Could you check a few things on this model? Use its own coordinates, in mm. A direction names the side the tool comes from. Give positions to 0.01 mm unless a question says otherwise; leave off trailing zeros. Loops run counter-clockwise (first coordinate to the right, second up) from the corner with the lowest first, then second, coordinate; pieces in that order, holes last. Notation, with made-up numbers: M 46,43 L 61,43 A13 ccw 61,58 Z; hole C -13,75 d1. An arc over 180 degrees is marked long. Return JSON: item names as keys, results as strings. Group by question number.
1. For pin 1 (5 mm diameter, centred on x = 4.5, z = 17, fed in from +Y); pin 2 (6 mm diameter, centred on x = -10.65, y = 5.23, fed in from +Z); pin 3 (6 mm diameter, centred on x = -4.5, z = 4, fed in from -Y); pin 4 (1 mm diameter, centred on y = 3, z = 2.5, fed in from -X), each with a flat end and sliding along its axis, tell me the tip position at first contact or that it passes through.
2. For faces 5 (the flat face through (-11, 5, 10.16)), 6 (the flat face through (15, 4, 3.6)), 7 (the flat face through (3, 7.85, 10)), 8 (the flat face through (13.3, 4, 3)), 9 (the flat face through (-10, -7.85, 7)), which set-ups out of +Z, -Z, +X, -X, +Y, -Y let a thin tool reach every point of the face, with its end or its side?
3. If we section it at D-D (x = 6.5): Write out the boundary of the cut face in (y, z).
4. If we section it at C-C (z = 6.5): Write out the boundary of the cut face in (x, y).
5. If we section it at A-A (y = 10.9): Write out the boundary of the cut face in (x, z).
6. If we mould it in two halves opening along X, with no side actions, what happens to faces 1 (the flat face through (-17, 0, 1)), 2 (the flat face through (0, -13.25, 1)), 3 (the flat face through (17, 0, 1)), 4 (the flat face through (-6.2, 0, 10))? For each: +X half, -X half, draft (parallel to the pull), parting line (faces both ways), or undercut.
7. If we section it at B-B (x = 14.4): Write out the boundary of the cut face in (y, z).
8. Please list where these lines run through material, in increasing order: line 1 (Y direction, x = 14.4, z = 1.15); line 2 (Y direction, x = -10.65, z = 11); line 3 (X direction, y = 5.25, z = 10.75).
Autodesk Inventor part; units mm, degrees
ref_plane "YZ Plane" through (0, 0, 0) normal (1, 0, 0) x (0, 1, 0)
ref_plane "XZ Plane" through (0, 0, 0) normal (0, 1, 0) x (-1, 0, 0)
ref_plane "XY Plane" through (0, 0, 0) normal (0, 0, 1) x (1, 0, 0)
sketch "스케치1" plane through (0, 0, 0) normal (0, 0, 1) x (1, 0, 0)
  line L0 (-17, 13.25) -> (17, 13.25)
  line L1 (17, 13.25) -> (17, -13.25)
  line L2 (17, -13.25) -> (-17, -13.25)
  line L3 (-17, -13.25) -> (-17, 13.25)
  line L4 (-17, 13.25) -> (17, -13.25) construction
  line L5 (17, 13.25) -> (-17, -13.25) construction
  circle A0 centre (14.4, 10.9) radius 1.4
  line L6 (0, 0) -> (4.1971, 0)
  line L7 (0, 0) -> (0, 5.4603)
  circle A1 centre (-14.4, 10.9) radius 1.4
  circle A2 centre (14.4, -10.9) radius 1.4
  circle A3 centre (-14.4, -10.9) radius 1.4
  dimension "d0" = 34
  dimension "d1" = 26.5
  dimension "d2" = 28.8
  dimension "d3" = 2.8
  dimension "d4" = 21.8
extrude "돌출1" add sketch "스케치1" along normal blind 1.6
sketch "스케치2" plane through (0, 0, 1.6) normal (0, 0, 1) x (1, 0, 0)
  line L0 (12.6, -7.85) -> (-6.2, -7.85)
  line L1 (-6.2, -7.85) -> (-6.2, 7.85)
  line L2 (-6.2, 7.85) -> (12.6, 7.85)
  line L3 (12.6, 7.85) -> (12.6, -7.85)
  line L4 (12.6, -7.85) -> (-6.2, 7.85) construction
  line L5 (-6.2, -7.85) -> (12.6, 7.85) construction
  line L6 (17, -13.25) -> (17, 13.25)
  point P0 (0, 0)
  point P1 (3.2, 0)
  dimension "d7" = 15.7
  dimension "d8" = 18.8
  dimension "d9" = 4.4
extrude "돌출2" add sketch "스케치2" along normal blind 17.2
sketch "스케치3" plane through (-6.2, 7.85, 1.6) normal (0, 1, 0) x (1, 0, 0)
  line L0 (0, 0) -> (18.8, 0)
  line L1 (0, 0) -> (-1.75, 0)
  line L2 (-1.75, 0) -> (-1.75, -6.84)
  line L3 (-1.75, -6.84) -> (0, -6.84)
  line L4 (0, -6.84) -> (0, 0)
  line L5 (-1.75, 0) -> (-7.75, 0)
  line L6 (-7.75, 0) -> (-7.75, -10.1)
  line L7 (-7.75, -10.1) -> (-1.75, -10.1)
  line L8 (-1.75, -10.1) -> (-1.75, 0)
  line L9 (-7.15, -10.1) -> (-7.75, -6.4)
  line L10 (-0.1, -6.84) -> (-0.1, 0)
  line L11 (23.2, 0) -> (-10.8, 0)
  point P0 (6.2, 1.6)
  point P1 (-1.75, -6.84)
  dimension "d12" = 1.75
  dimension "d13" = 6.84
  dimension "d14" = 6
  dimension "d15" = 10.1
  dimension "d16" = 0.6
  dimension "d17" = 3.7
  dimension "d20" = 0.1
extrude "돌출3" add sketch "스케치3" against normal blind 15.7 contours L10 L3 L2 L1 | L2 L8 L7 L9 L6 L5
sketch "스케치4" plane through (-13.35, 7.85, 11.7) normal (0, 0, 1) x (1, 0, 0)
  line L0 (0, 0) -> (5.4, 0)
  line L1 (0, 0) -> (0, -15.7)
  line L2 (5.4, -15.7) -> (0, -15.7)
  line L3 (5.4, 0) -> (5.4, -15.7)
  line L4 (5.4, 0) -> (5.4, -15.7)
  line L5 (5.4, -7.85) -> (0, -7.85)
  circle A0 centre (2.7, -7.85) radius 1.9
  circle A1 centre (2.7, -13.0833) radius 1.9
  circle A2 centre (2.7, -2.6167) radius 1.9
  circle A3 centre (2.7, -7.85) radius 1.9
  point P0 (13.35, -7.85)
  dimension "d21" = 3.8
  dimension "d24" = 5.2333
  dimension "d27" = 5.2333
extrude "돌출4" cut sketch "스케치4" against normal blind 1.54 contours A0 L5 | L5 A0 | A1 | A2
sketch "스케치5" plane through (0, 0, 1.6) normal (0, 0, 1) x (1, 0, 0)
  line L0 (15.8, 7.85) -> (13.3, 7.85)
  line L1 (13.3, 7.85) -> (13.3, 0.4)
  line L2 (13.3, 0.4) -> (15.8, 0.4)
  line L3 (15.8, 0.4) -> (15.8, 7.85)
  line L4 (17, -13.25) -> (17, 13.25)
  point P0 (0, 0)
  dimension "d32" = 2.5
  dimension "d33" = 7.45
  dimension "d34" = 1.2
extrude "돌출5" add sketch "스케치5" along normal blind 2
chamfer "모따기1" distance 0.5 angle 45 4 edges at (15.8, 7.85, 2.6) (15.8, 0.4, 2.6) (13.3, 7.85, 2.6) (13.3, 0.4, 2.6)
properties part number "릴레이모듈"
Answer:
{
 "1": {"pin 1": "stops at y = 7.85", "pin 2": "stops at z = 11.7", "pin 3": "stops at y = -13.25", "pin 4": "stops at x = -13.95"},
 "2": {"face 5": "+Z", "face 6": "+Z, +X, +Y, -Y", "face 7": "+Z, +X, -X, +Y", "face 8": "+Z, +Y, -Y", "face 9": "+Z, +X, -X, -Y"},
 "3": {"outline": "M -13.25,0 L 13.25,0 L 13.25,1.6 L 7.85,1.6 L 7.85,18.8 L -7.85,18.8 L -7.85,1.6 L -13.25,1.6 Z"},
 "4": {"outline": "M -13.95,-7.85 L -6.3,-7.85 L -6.3,7.85 L -13.95,7.85 Z; M -6.2,-7.85 L 12.6,-7.85 L 12.6,7.85 L -6.2,7.85 Z"},
 "5": {"outline": "M -17,0 L -15.8,0 L -15.8,1.6 L -17,1.6 Z; M -13,0 L 13,0 L 13,1.6 L -13,1.6 Z; M 15.8,0 L 17,0 L 17,1.6 L 15.8,1.6 Z"},
 "6": {"face 1": "-X half", "face 2": "draft", "face 3": "+X half", "face 4": "undercut"},
 "7": {"outline": "M -13.25,0 L -12.3,0 L -12.3,1.6 L -13.25,1.6 Z; M -9.5,0 L 9.5,0 L 9.5,1.6 L 7.85,1.6 L 7.85,3.6 L 0.4,3.6 L 0.4,1.6 L -9.5,1.6 Z; M 12.3,0 L 13.25,0 L 13.25,1.6 L 12.3,1.6 Z"},
 "8": {"line 1": "y = -13.25 to -12.3, -9.5 to 9.5, 12.3 to 13.25", "line 2": "y = -7.85 to -7.13, -3.33 to -1.9, 1.9 to 3.33, 7.13 to 7.85", "line 3": "x = -13.5 to -12.55, -8.75 to -7.95, -6.2 to 12.6"}
}
